from build123d import *

# Parameters (mm, degrees)
SKETCH1_R               = 88.9
BOSS_EXTRUDE1_DEPTH     = 76.2
FILLET1_R               = 25.4
FILLET2_R               = 25.4
CUT_EXTRUDE1_DEPTH      = 148.013128726
CUT_EXTRUDE1_DEPTH_BACK = 148.013128726
SKETCH2_R               = 17.78


with BuildPart() as part:
    # Sketch1 → Boss-Extrude1 (new body)
    with BuildSketch(Plane(origin=(0, 0, 0), x_dir=(0, 0, -1), z_dir=(1, 0, 0))):
        with Locations(Location((0, 0, 0), (0, 0, 180))):
            Circle(SKETCH1_R)
    extrude(amount=BOSS_EXTRUDE1_DEPTH)

    # Fillet1
    fillet1_edges = [part.edges().sort_by_distance(p)[0] for p in [
        (76.2, 0, -88.9),
    ]]
    fillet(fillet1_edges, radius=FILLET1_R)

    # Fillet2
    fillet2_edges = [part.edges().sort_by_distance(p)[0] for p in [
        (0, 0, -88.9),
    ]]
    fillet(fillet2_edges, radius=FILLET2_R)

    # Sketch2 → Cut-Extrude1 (cut, two sides: drawn at the far end of the back side and taken through both)
    with BuildSketch(Plane.ZY.offset(-CUT_EXTRUDE1_DEPTH_BACK)):
        Circle(SKETCH2_R)
    extrude(amount=CUT_EXTRUDE1_DEPTH + CUT_EXTRUDE1_DEPTH_BACK, mode=Mode.SUBTRACT)


solid = part.part
Geometry check sheet. Reference: the model listing, model coordinates, mm. Round coordinates to 2 decimals unless told otherwise and drop trailing zeros. Write each loop counter-clockwise with the first axis right and the second up, starting at its lowest first coordinate (ties: lowest second). Pieces come first, ordered by that corner, then holes. Notation, with made-up numbers: (12, 75) -> (21, 75) arc R6 cw to (21, 82) -> close; hole circle Ø8 at (-26, -8.5). An arc over 180 degrees is marked (long way). One line per item, written item: value. Start each with the question number.
(1) Draft check along Z on faces 1 (the cylindrical face through (38.63, -17.36, -3.85)), 2 (the cylindrical face through (37.922, -60.083, -65.523)), 3 (the flat face through (0, 13, 13)). Enter one of: +Z half, -Z half, draft (parallel to the pull), parting line (faces both ways), or undercut.
(2) Cross-section at A-A, the plane z = 0. Record the cut outline in (x, y).
(3) Go/stop test with flat-tipped pins: pin 1 Ø12 at (y, z) = (-68, -38) entering from +X; pin 2 Ø1.5 at (x, z) = (18.5, -40) entering from +Y (3 decimals); pin 3 Ø2 at (y, z) = (56, 65) entering from +X. Record where each tip stops, or that it passes through.
(4) Scan lines: line 1 (Y direction, x = 29, z = 0); line 2 (Z direction, x = 67, y = 12); line 3 (Y direction, x = 67.5, z = -15). Record each from-to range of solid material in increasing order. Write a range as [from, to].
(5) Cross-section at C-C, the plane x = 44. Record the cut outline in (y, z), and give its area (3 significant figures).
(6) Cross-section at D-D, the plane x = 64. Record the cut outline in (y, z).
Answer:
1. face 1: undercut
1. face 2: parting line
1. face 3: draft
2. outline: (0, -63.5) arc R25.4 ccw to (25.4, -88.9) -> (50.8, -88.9) arc R25.4 ccw to (76.2, -63.5) -> (76.2, -17.78) -> (0, -17.78) -> close; (0, 17.78) -> (76.2, 17.78) -> (76.2, 63.5) arc R25.4 ccw to (50.8, 88.9) -> (25.4, 88.9) arc R25.4 ccw to (0, 63.5) -> close
3. pin 1: x = 74.77
3. pin 2: y = 78.765
3. pin 3: x = 64.64
4. line 1: [-88.9, -17.78], [17.78, 88.9]
4. line 2: [-82.19, -13.12], [13.12, 82.19]
4. line 3: [-81.27, -9.55], [9.55, 81.27]
5. outline: circle Ø177.8 at (0, 0); hole circle Ø35.56 at (0, 0)
5. area: 23,800 mm²
6. outline: circle Ø170.4 at (0, 0); hole circle Ø35.56 at (0, 0)
